Autodesk Inventor part; units mm, degrees
ref_plane "YZ Plane" through (0, 0, 0) normal (1, 0, 0) x (0, 1, 0)
ref_plane "XZ Plane" through (0, 0, 0) normal (0, 1, 0) x (-1, 0, 0)
ref_plane "XY Plane" through (0, 0, 0) normal (0, 0, 1) x (1, 0, 0)
sketch "Sketch2" plane through (0, 0, 0) normal (0, 1, 0) x (-1, 0, 0)
  line L0 (-30.2, -84) -> (30.2, -84)
  line L1 (30.2, -84) -> (30.2, 84)
  line L2 (30.2, 84) -> (-30.2, 84)
  line L3 (-30.2, 84) -> (-30.2, -84)
  line L4 (-30.2, -84) -> (30.2, 84) construction
  line L5 (30.2, -84) -> (-30.2, 84) construction
  point P0 (0, 0)
  dimension "d0" = 60.4
  dimension "d1" = 168
extrude "Extrusion1" add sketch "Sketch2" along normal blind 3
sketch "Sketch3" plane through (0, 3, 0) normal (0, 1, 0) x (1, 0, 0)
  line L0 (27.2, 81) -> (-27.2, 81)
  line L1 (-27.2, 81) -> (-27.2, -81)
  line L2 (-27.2, -81) -> (27.2, -81)
  line L3 (27.2, -81) -> (27.2, 81)
  line L4 (27.2, 81) -> (-27.2, -81) construction
  line L5 (-27.2, 81) -> (27.2, -81) construction
  line L6 (-30.2, 84) -> (-30.2, -84)
  line L7 (-30.2, -84) -> (30.2, -84)
  line L8 (24.2, 78) -> (-24.2, 78)
  line L9 (-24.2, 78) -> (-24.2, -78)
  line L10 (-24.2, -78) -> (24.2, -78)
  line L11 (24.2, -78) -> (24.2, 78)
  line L12 (24.2, 78) -> (-24.2, -78) construction
  line L13 (-24.2, 78) -> (24.2, -78) construction
  point P0 (0, 0)
  dimension "d4" = 3
  dimension "d5" = 3
  dimension "d6" = 3
  dimension "d7" = 3
extrude "Extrusion2" add sketch "Sketch3" along normal blind 30
fillet "Fillet1" radius 2 8 edges at (27.2, 18, 81) (-27.2, 18, 81) (-30.2, 1.5, 84) (30.2, 1.5, 84) (27.2, 18, -81) (-27.2, 18, -81) (30.2, 1.5, -84) (-30.2, 1.5, -84)
sketch "Sketch10" plane through (0, 3, 0) normal (0, 1, 0) x (1, 0, 0)
  line L0 (24.2, 78) -> (-24.2, 78)
  line L1 (-24.2, 78) -> (-24.2, -78)
  line L2 (-24.2, -78) -> (24.2, -78)
  line L3 (24.2, -78) -> (24.2, 78)
  line L4 (-24.2, -78) -> (24.2, -78)
  line L5 (24.2, -78) -> (24.2, -73.8)
  line L6 (24.2, -73.8) -> (-24.2, -73.8)
  line L7 (-24.2, -73.8) -> (-24.2, -78)
  line L8 (-24.2, -73.8) -> (24.2, -73.8)
  line L9 (24.2, -73.8) -> (24.2, 22.3)
  line L10 (24.2, 22.3) -> (-24.2, 22.3)
  line L11 (-24.2, 22.3) -> (-24.2, -73.8)
  line L12 (-24.2, 22.3) -> (24.2, 22.3)
  line L13 (24.2, 22.3) -> (24.2, 26.3)
  line L14 (24.2, 26.3) -> (-24.2, 26.3)
  line L15 (-24.2, 26.3) -> (-24.2, 22.3)
  point P0 (0, 0)
  point P1 (-24.2, 26.3)
  point P2 (-24.2, 22.3)
  dimension "d90" = 4.2
  dimension "d91" = 96.1
  dimension "d92" = 4
extrude "Extrusion9" add sketch "Sketch10" along normal blind 3 contours L3 L10 L1 L14 | L3 L2 L1 L6
sketch "Sketch11" plane through (0, 6, 0) normal (0, 1, 0) x (1, 0, 0)
  line L0 (-24.2, 22.3) -> (-24.2, 26.3)
  line L1 (-24.2, 22.3) -> (24.2, 22.3)
  line L2 (24.2, 26.3) -> (24.2, 22.3)
  line L3 (24.2, 26.3) -> (-24.2, 26.3)
  line L4 (-24.2, -78) -> (-24.2, -73.8)
  line L5 (24.2, -78) -> (-24.2, -78)
  line L6 (24.2, -73.8) -> (24.2, -78)
  line L7 (24.2, -73.8) -> (-24.2, -73.8)
  line L8 (24.2, 26.3) -> (-24.2, 26.3)
  line L9 (-24.2, 26.3) -> (24.2, 26.3)
  line L10 (24.2, 26.3) -> (24.2, 24.3)
  line L11 (24.2, 24.3) -> (-24.2, 24.3)
  line L12 (-24.2, 24.3) -> (-24.2, 26.3)
  line L13 (24.2, 26.3) -> (24.2, -78)
  line L14 (-24.2, -78) -> (24.2, -78)
  line L15 (24.2, -78) -> (24.2, -76)
  line L16 (24.2, -76) -> (-24.2, -76)
  line L17 (-24.2, -76) -> (-24.2, -78)
  line L18 (-24.2, 22.3) -> (-24.2, 26.3)
  line L19 (-24.2, 22.3) -> (24.2, 22.3)
  line L20 (24.2, 26.3) -> (-24.2, 26.3)
  line L21 (24.2, 26.3) -> (24.2, 22.3)
  point P0 (0, 0)
  point P1 (24.2, -72.6)
  point P2 (-24.2, 24.3)
  point P3 (-24.2, -76)
  point P4 (-24.2, -76)
  dimension "d95" = 2
  dimension "d120" = 2
extrude "Extrusion10" add sketch "Sketch11" along normal blind 1.6 contours L0 L3 L2 L11 | L6 L5 L4 L16
sketch "Sketch12" plane through (-25.2, 3, 81) normal (0, 0, 1) x (1, 0, 0)
  line L0 (-2, 30) -> (-2, 0)
  line L1 (0, 30) -> (50.4, 30)
  line L2 (-2, 30) -> (0, 30)
  line L3 (50.4, 30) -> (52.4, 30)
  line L4 (52.4, 0) -> (52.4, 30)
  line L5 (50.4, 0) -> (0, 0)
  line L6 (0, 0) -> (-2, 0)
  line L7 (52.4, 0) -> (50.4, 0)
  line L8 (15, 23.6) -> (23.06, 23.6)
  line L9 (23.06, 23.6) -> (23.06, 15)
  line L10 (23.06, 15) -> (15, 15)
  line L11 (15, 15) -> (15, 23.6)
  line L12 (27.34, 23.6) -> (35.4, 23.6)
  line L13 (35.4, 23.6) -> (35.4, 15)
  line L14 (35.4, 15) -> (27.34, 15)
  line L15 (27.34, 15) -> (27.34, 23.6)
  point P0 (25.2, -3)
  dimension "d116" = 8.06
  dimension "d117" = 8.6
  dimension "d118" = 15
  dimension "d119" = 17
  dimension "d121" = 8.06
  dimension "d122" = 8.6
  dimension "d123" = 15
  dimension "d124" = 17
extrude "Extrusion11" cut sketch "Sketch12" against normal blind 3 contours L8 L9 L10 L11 | L12 L13 L14 L15
sketch "Sketch13" plane through (0, 3, 0) normal (0, 1, 0) x (1, 0, 0)
  arc A0 (-28.2, 84) -> (-30.2, 82) centre (-28.2, 82) ccw
  line L0 (-30.2, 82) -> (-30.2, -82)
  arc A1 (-30.2, -82) -> (-28.2, -84) centre (-28.2, -82) ccw
  line L1 (-28.2, -84) -> (28.2, -84)
  arc A2 (28.2, -84) -> (30.2, -82) centre (28.2, -82) ccw
  line L2 (30.2, -82) -> (30.2, 82)
  arc A3 (30.2, 82) -> (28.2, 84) centre (28.2, 82) ccw
  line L3 (28.2, 84) -> (-28.2, 84)
  line L4 (-25.2, 81) -> (25.2, 81)
  arc A4 (27.2, 79) -> (25.2, 81) centre (25.2, 79) ccw
  line L5 (27.2, 79) -> (27.2, -79)
  arc A5 (25.2, -81) -> (27.2, -79) centre (25.2, -79) ccw
  line L6 (25.2, -81) -> (-25.2, -81)
  arc A6 (-27.2, -79) -> (-25.2, -81) centre (-25.2, -79) ccw
  line L7 (-27.2, -79) -> (-27.2, 79)
  arc A7 (-25.2, 81) -> (-27.2, 79) centre (-25.2, 79) ccw
  point P0 (0, 0)
extrude "Extrusion12" cut sketch "Sketch13" against normal blind 3
sketch "Sketch14" plane through (25.2, 33, -81) normal (0, 0, -1) x (-1, 0, 0)
  line L0 (1, -10) -> (49.4, -10)
  line L1 (49.4, -10) -> (49.4, -19.6)
  line L2 (49.4, -19.6) -> (1, -19.6)
  line L3 (1, -19.6) -> (1, -10)
  line L4 (52.4, -33) -> (52.4, 0)
  line L5 (-2, 0) -> (-2, -33)
  line L6 (50.4, 0) -> (50.4, -33)
  line L7 (50.4, -33) -> (0, -33)
  point P0 (25.2, -33)
  point P1 (50.4, -16.5)
  point P2 (49.4, -14.8)
  dimension "d127" = 9.6
  dimension "d128" = 3
  dimension "d129" = 3
  dimension "d140" = 23
extrude "Extrusion13" add sketch "Sketch14" along normal blind 6
sketch "Sketch15" plane through (-24.2, 13.4, -81) normal (-1, 0, 0) x (0, 0, 1)
  line L0 (0, 9.6) -> (-6, 9.6)
  line L1 (0, 9.6) -> (-3.4, 9.6)
  line L2 (-3.4, 9.6) -> (-3.4, 6.6)
  line L3 (-3.4, 6.6) -> (0, 6.6)
  line L4 (0, 6.6) -> (0, 9.6)
  line L5 (0, 9.6) -> (0, 0)
  line L6 (0, 9.6) -> (-6, 9.6)
  line L7 (-6, 0) -> (-6, 9.6)
  line L8 (0, 0) -> (-6, 0)
  line L9 (0, 0) -> (-3.4, 0)
  line L10 (-3.4, 0) -> (-3.4, 3)
  line L11 (-3.4, 3) -> (0, 3)
  line L12 (0, 3) -> (0, 0)
  point P0 (81, -13.4)
  point P1 (-3.4, 0)
  dimension "d133" = 3.4
  dimension "d134" = 3
  dimension "d135" = 3.4
  dimension "d136" = 3
extrude "Extrusion14" cut sketch "Sketch15" against normal up to surface (48.4 mm away) contours L4 L3 L2 L0 | L5 L8 L10 L11
fillet "Fillet8" radius 1 18 edges at (0, 23, -87) (0, 23, -84.4) (0, 13.4, -87) (0, 13.4, -84.4) (-24.2, 14.9, -84.4) (-24.2, 18.2, -87) (-24.2, 21.5, -84.4) (-24.2, 23, -85.7) (-24.2, 13.4, -85.7) (-24.2, 16.4, -82.7) (-24.2, 20, -82.7) (24.2, 20, -82.7) (24.2, 16.4, -82.7) (24.2, 14.9, -84.4) (24.2, 21.5, -84.4) (24.2, 23, -85.7) (24.2, 18.2, -87) (24.2, 13.4, -85.7)
sketch "Sketch16" plane through (-27.2, 0, -79) normal (-1, 0, 0) x (0, 0, 1)
  line L0 (147, 22.8) -> (134.9, 22.8)
  line L1 (134.9, 22.8) -> (134.9, 18)
  line L2 (134.9, 18) -> (147, 18)
  line L3 (147, 18) -> (147, 22.8)
  line L4 (160, 3) -> (160, 33)
  line L5 (152, 0) -> (0, 0)
  point P0 (79, 0)
  point P1 (154, 0)
  dimension "d141" = 12.1
  dimension "d142" = 4.8
  dimension "d143" = 13
  dimension "d144" = 18
extrude "Extrusion15" cut sketch "Sketch16" against normal through all
sketch "Sketch17" plane through (0, 33, 0) normal (0, 1, 0) x (1, 0, 0)
  arc A0 (-25.2, 81) -> (-27.2, 79) centre (-25.2, 79) ccw
  line L0 (-27.2, 79) -> (-27.2, -79)
  arc A1 (-27.2, -79) -> (-25.2, -81) centre (-25.2, -79) ccw
  line L1 (-25.2, -81) -> (25.2, -81)
  arc A2 (25.2, -81) -> (27.2, -79) centre (25.2, -79) ccw
  line L2 (27.2, -79) -> (27.2, 79)
  arc A3 (27.2, 79) -> (25.2, 81) centre (25.2, 79) ccw
  line L3 (25.2, 81) -> (-25.2, 81)
  line L4 (24.2, 78) -> (24.2, -78)
  line L5 (24.2, -78) -> (-24.2, -78)
  line L6 (-24.2, -78) -> (-24.2, 78)
  line L7 (-24.2, 78) -> (24.2, 78)
  line L8 (-26.2, 20) -> (-24.2, 20)
  line L9 (-24.2, 20) -> (-24.2, 16.6)
  line L10 (-24.2, 16.6) -> (-26.2, 16.6)
  line L11 (-26.2, 16.6) -> (-26.2, 20)
  line L12 (-24.2, -0.56) -> (-26.2, -0.56)
  line L13 (-26.2, -0.56) -> (-26.2, -3.96)
  line L14 (-26.2, -3.96) -> (-24.2, -3.96)
  line L15 (-24.2, -3.96) -> (-24.2, -0.56)
  line L16 (-24.2, 22.3) -> (-24.2, 26.3)
  line L17 (-24.2, -21.12) -> (-26.2, -21.12)
  line L18 (-26.2, -21.12) -> (-26.2, -24.52)
  line L19 (-26.2, -24.52) -> (-24.2, -24.52)
  line L20 (-24.2, -24.52) -> (-24.2, -21.12)
  line L21 (24.2, 20) -> (26.2, 20)
  line L22 (26.2, 20) -> (26.2, 16.6)
  line L23 (26.2, 16.6) -> (24.2, 16.6)
  line L24 (24.2, 16.6) -> (24.2, 20)
  line L25 (24.2, -0.56) -> (26.2, -0.56)
  line L26 (26.2, -0.56) -> (26.2, -3.96)
  line L27 (26.2, -3.96) -> (24.2, -3.96)
  line L28 (24.2, -3.96) -> (24.2, -0.56)
  line L29 (24.2, -21.12) -> (26.2, -21.12)
  line L30 (26.2, -21.12) -> (26.2, -24.52)
  line L31 (26.2, -24.52) -> (24.2, -24.52)
  line L32 (24.2, -24.52) -> (24.2, -21.12)
  point P0 (0, 0)
  point P1 (-24.2, 16.6)
  point P2 (-24.2, -73.8)
  point P3 (24.2, 16.6)
  point P4 (24.2, -3.96)
  point P5 (24.2, -24.52)
  point P6 (-24.2, -24.52)
  point P7 (-24.2, -21.12)
  point P8 (-24.2, -3.96)
  dimension "d147" = 2
  dimension "d148" = 3.4
  dimension "d149" = 61
  dimension "d150" = 0
  dimension "d153" = 2
  dimension "d154" = 3.4
  dimension "d155" = 20.56
  dimension "d156" = 2
  dimension "d157" = 3.4
  dimension "d158" = 20.56
  dimension "d159" = 2
  dimension "d160" = 3.4
  dimension "d161" = 2
  dimension "d162" = 3.4
  dimension "d163" = 2
  dimension "d164" = 3.4
  dimension "d165" = 20.56
  dimension "d166" = 20.56
  dimension "d167" = 61
extrude "Extrusion16" cut sketch "Sketch17" against normal blind 3.2 contours L21 L22 L23 L4 | L25 L26 L27 L4 | L6 L10 L11 L8 | L29 L30 L31 L4 | L6 L14 L13 L12 | L6 L19 L18 L17
sketch "Sketch18" plane through (0, 33, 0) normal (0, 1, 0) x (1, 0, 0)
  line L0 (24.2, -21.12) -> (26.2, -21.12)
  line L1 (26.2, -21.12) -> (26.2, -24.52)
  line L2 (26.2, -24.52) -> (24.2, -24.52)
  line L3 (24.2, -24.52) -> (24.2, -78)
  line L4 (24.2, -78) -> (-24.2, -78)
  line L5 (-24.2, -78) -> (-24.2, -24.52)
  line L6 (-24.2, -24.52) -> (-26.2, -24.52)
  line L7 (-26.2, -24.52) -> (-26.2, -21.12)
  line L8 (-26.2, -21.12) -> (-24.2, -21.12)
  line L9 (-24.2, -21.12) -> (-24.2, -3.96)
  line L10 (-24.2, -3.96) -> (-26.2, -3.96)
  line L11 (-26.2, -3.96) -> (-26.2, -0.56)
  line L12 (-26.2, -0.56) -> (-24.2, -0.56)
  line L13 (-24.2, -0.56) -> (-24.2, 16.6)
  line L14 (-24.2, 16.6) -> (-26.2, 16.6)
  line L15 (-26.2, 16.6) -> (-26.2, 20)
  line L16 (-26.2, 20) -> (-24.2, 20)
  line L17 (-24.2, 20) -> (-24.2, 78)
  line L18 (-24.2, 78) -> (24.2, 78)
  line L19 (24.2, 78) -> (24.2, 20)
  line L20 (24.2, 20) -> (26.2, 20)
  line L21 (26.2, 20) -> (26.2, 16.6)
  line L22 (26.2, 16.6) -> (24.2, 16.6)
  line L23 (24.2, 16.6) -> (24.2, -0.56)
  line L24 (24.2, -0.56) -> (26.2, -0.56)
  line L25 (26.2, -0.56) -> (26.2, -3.96)
  line L26 (26.2, -3.96) -> (24.2, -3.96)
  line L27 (24.2, -3.96) -> (24.2, -21.12)
  arc A0 (-25.2, 81) -> (-27.2, 79) centre (-25.2, 79) ccw
  line L28 (-27.2, 79) -> (-27.2, -79)
  arc A1 (-27.2, -79) -> (-25.2, -81) centre (-25.2, -79) ccw
  line L29 (-25.2, -81) -> (25.2, -81)
  arc A2 (25.2, -81) -> (27.2, -79) centre (25.2, -79) ccw
  line L30 (27.2, -79) -> (27.2, 79)
  arc A3 (27.2, 79) -> (25.2, 81) centre (25.2, 79) ccw
  line L31 (25.2, 81) -> (-25.2, 81)
  line L32 (27.2, 31.5) -> (-27.2, 31.5)
  line L33 (-27.2, 31.5) -> (-27.2, 181.5)
  line L34 (-27.2, 181.5) -> (27.2, 181.5)
  line L35 (27.2, 181.5) -> (27.2, 31.5)
  line L36 (24.2, -55.9) -> (27.2, -55.9)
  line L37 (24.2, 26.5) -> (-24.2, 26.5)
  point P0 (0, 0)
  point P1 (27.2, 79)
  point P2 (24.2, 26.3)
  point P3 (-24.2, 26.3)
  dimension "d168" = 150
  dimension "d179" = 5
extrude "Extrusion17" cut sketch "Sketch18" against normal through all contours L32 L19 L18 L17 L28 A0 L31 A3 L30 | A3 L31 A0 L33 L34 L35 | L32 L17 L18 L19
sketch "Sketch19" plane through (0, 0, 0) normal (0, -1, 0) x (1, 0, 0)
  line L0 (-27.2, -31.5) -> (27.2, -31.5)
  line L1 (27.2, -31.5) -> (27.2, 79)
  arc A0 (27.2, 79) -> (25.2, 81) centre (25.2, 79) ccw
  line L2 (25.2, 81) -> (-25.2, 81)
  arc A1 (-25.2, 81) -> (-27.2, 79) centre (-25.2, 79) ccw
  line L3 (-27.2, 79) -> (-27.2, -31.5)
  point P0 (0, 0)
extrude "Extrusion18" cut sketch "Sketch19" against normal blind 3
equation "\"d167\" = d149"
properties part number "module_switch" material "PC/ABS Plastic"
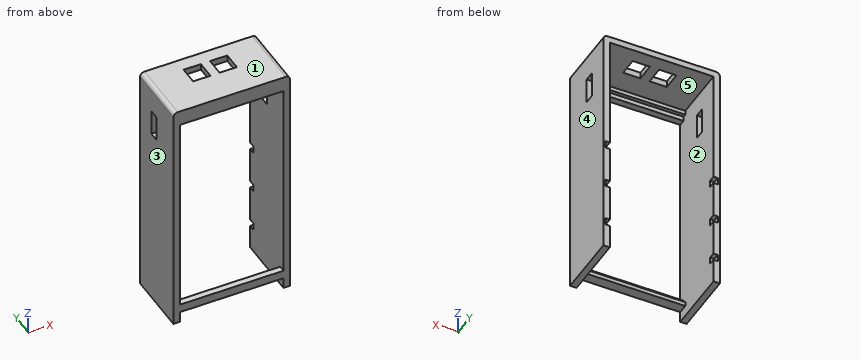
Work out the finished part from the listing and answer in its coordinate system (mm). Face numbers are marked on the shaded views. A direction names the side the tool comes from. Give positions to 0.01 mm unless a question says otherwise; leave off trailing zeros. Loops run counter-clockwise (first coordinate to the right, second up) from the corner with the lowest first, then second, coordinate; pieces in that order, holes last. Notation, with made-up numbers: (-10, 18.25) - (31, 18.25) arc R16 cw to (31, 35.25) - close; hole circle Ø7 at (54.25, -26). An arc over 180 degrees is marked (long way). Use CSV: the item, a comma, the result in double quotes. Start each with the question number.
(1) Find the intervals of material crossed by L1, parallel to X at y = 23.25, z = 46; L2, parallel to Z at x = -20.5, y = 26.5; L3, parallel to Z at x = -24, y = 6.75, in increasing order.
(2) Determine the mould class of the marked faces 1, 2 and 3 for opening direction X: released by +X, released by -X, zero draft, split by the parting line, or undercut.
(3) Find section A-A, the plane y = 20.75. Determine the outline of the cut face in (x, z).
(4) Each of these flat-tipped pins is pushed along its axis until it touches: pin 1 (12 mm diameter, centred on x = 3.5, y = 15.5, fed in from -Z); pin 2 (0.6 mm diameter, centred on x = -9, z = -23.5, fed in from +Y); pin 3 (0.6 mm diameter, centred on x = 25, z = 1.5, fed in from +Y). Where does it stop, or does it pass through?
(5) A tool of negligible diameter and unlimited length cuts with its end or side. For the marked faces 4 and 5, from which of +Z, -Z, +X, -X, +Y, -Y can it reach the whole face along a straight path? Write none if from no direction.
(6) Find section C-C, the plane x = -13. Determine the outline of the cut face in (y, z).
(7) Find section B-B, the plane z = 6.5. Determine the outline of the cut face in (x, y).
(8) Find section D-D, the plane x = 8.5. Determine the outline of the cut face in (y, z), plus the area to 3 significant figures.
Results found:
1,L1,"-27.2 to -24.2, 24.2 to 27.2"
1,L2,"78 to 81"
1,L3,"-26.3 to -24.3, 76 to 81"
2,face 1,"zero draft"
2,face 2,"undercut"
2,face 3,"released by -X"
3,outline,"(-27.2, -31.5) - (-24.2, -31.5) - (-24.2, 55.9) - (-27.2, 55.9) - close; (-27.2, 68) - (-24.2, 68) - (-24.2, 78) - (-10.2, 78) - (-10.2, 81) - (-25.2, 81) arc R2 ccw to (-27.2, 79) - close; (-2.14, 78) - (2.14, 78) - (2.14, 81) - (-2.14, 81) - close; (10.2, 78) - (24.2, 78) - (24.2, 68) - (27.2, 68) - (27.2, 79) arc R2 ccw to (25.2, 81) - (10.2, 81) - close; (24.2, -31.5) - (27.2, -31.5) - (27.2, 55.9) - (24.2, 55.9) - close"
4,pin 1,"z = 78"
4,pin 2,"y = 6"
4,pin 3,"y = 29.8"
5,face 4,"+Z, -Z, +X, +Y, -Y"
5,face 5,"-Z, +Y"
6,outline,"(3, -26.3) - (7.6, -26.3) - (7.6, -24.3) - (6, -24.3) - (6, -22.3) - (3, -22.3) - close; (3, 73.8) - (6, 73.8) - (6, 76) - (7.6, 76) - (7.6, 78) - (33, 78) - (33, 81) - (3, 81) - close"
7,outline,"(-27.2, 3) - (-24.2, 3) - (-24.2, 33) - (-27.2, 33) - close; (24.2, 3) - (27.2, 3) - (27.2, 33) - (24.2, 33) - close"
8,outline,"(3, -26.3) - (7.6, -26.3) - (7.6, -24.3) - (6, -24.3) - (6, -22.3) - (3, -22.3) - close; (3, 73.8) - (6, 73.8) - (6, 76) - (7.6, 76) - (7.6, 78) - (18, 78) - (18, 81) - (3, 81) - close; (26.6, 78) - (33, 78) - (33, 81) - (26.6, 81) - close"
8,area,"95.2 mm^2"
